Part model, mm, in its own coordinate system. Round coordinates to 2 decimals unless told otherwise and drop trailing zeros. Loops run counter-clockwise (first coordinate to the right, second up) from the corner with the lowest first, then second, coordinate; pieces in that order, holes last. Notation, with made-up numbers: M 87,-29 L 99,-29 A30 ccw 99,6 Z; hole C -11,38.5 d6. An arc over 180 degrees is marked long. Put each result on its own line as item: value. Start each with the question number.
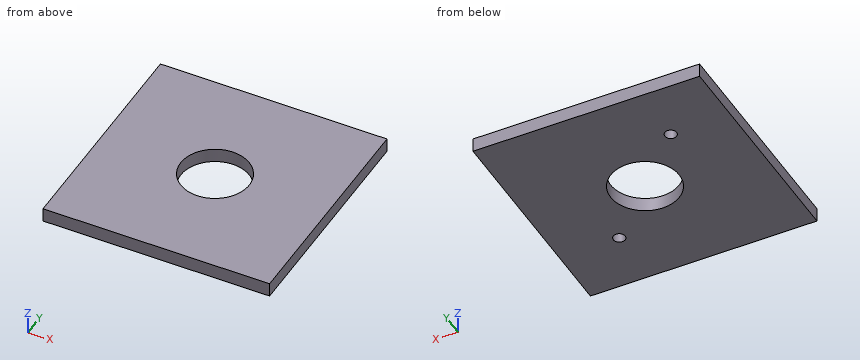
```python
from build123d import *

# Parameters (mm, degrees)
SKETCH1_W           = 304.8
SKETCH1_H           = 304.8
SKETCH1_R           = 46.0375
BOSS_EXTRUDE1_DEPTH = 19.05
SKETCH2_R           = 7.9375
CUT_EXTRUDE1_DEPTH  = 15.875


with BuildPart() as part:
    # Sketch1 → Boss-Extrude1 (new body)
    with BuildSketch(Plane.XY):
        Rectangle(SKETCH1_W, SKETCH1_H)
        with Locations(Location((0, 0, 0), (0, 0, 180))):
            Circle(SKETCH1_R, mode=Mode.SUBTRACT)
    extrude(amount=BOSS_EXTRUDE1_DEPTH)

    # Sketch2 → Cut-Extrude1 (cut)
    with BuildSketch(Plane.XY):
        with Locations(Location((-71.842048969, 71.842048969, 0), (0, 0, 180))):
            Circle(SKETCH2_R)
        with Locations(Location((71.842048969, -71.842048969, 0), (0, 0, 180))):
            Circle(SKETCH2_R)
    extrude(amount=CUT_EXTRUDE1_DEPTH, mode=Mode.SUBTRACT)


solid = part.part
```
1. Drop a flat-ended pin along its axis: pin 1 (5 mm diameter, centred on x = -75.5, y = 72.5, fed in from -Z) (3 decimals). Give the stop position or say it passes through.
2. Wall check: L1, parallel to X at y = 72.5, z = 12; L2, parallel to Y at x = 0, z = 12.5; L3, parallel to Y at x = 31, z = 5.25. Give the ranges that are in metal, low to high.
3. Cut at A-A, the plane x = 0. Give the cut face in (y, z), and give its area (3 significant figures).
4. Cut at C-C, the plane z = 11.25. Give the cut face in (x, y) (1 decimal).
Results list:
1. pin 1: stops at z = 15.875
2. L1: x = -152.4 to -79.75, -63.93 to 152.4
2. L2: y = -152.4 to -46.04, 46.04 to 152.4
2. L3: y = -152.4 to -34.04, 34.04 to 152.4
3. outline: M -152.4,0 L -46.04,0 L -46.04,19.05 L -152.4,19.05 Z; M 46.04,0 L 152.4,0 L 152.4,19.05 L 46.04,19.05 Z
3. area: 4,050 mm^2
4. outline: M -152.4,-152.4 L 152.4,-152.4 L 152.4,152.4 L -152.4,152.4 Z; hole C -71.8,71.8 d15.9; hole C 0,0 d92.1; hole C 71.8,-71.8 d15.9
